Input: part model. Units: mm. Frame: model coordinates. A direction names the side the tool comes from. Coordinates: 2 decimals unless noted, no trailing zeros. Write each loop counter-clockwise with the first axis right and the second up, starting at its lowest first coordinate (ties: lowest second). Pieces come first, ordered by that corner, then holes. Notation, with made-up numbers: (39.25, -34) - (93.25, -34) arc R19 ccw to (93.25, 2) - close; hole circle Ø8 at (15.25, 9.5). An arc over 180 degrees is marked (long way). One line per question, with ' | ' between items. Start each with the question number.
1) Section query C-C on x = -17. Return loops of the section in (y, z), and give its area (3 significant figures).
2) First-contact query: P1, Ø14.5, axis at y = -453, z = 0, coming from the +X side. Flat tip, straight axial feed; report the tip coordinate or a pass-through.
3) Section query B-B on y = -453. Return loops of the section in (x, z), and give its area (3 significant figures).
4) Draft query along Y for faces 1 (the cylindrical face through (-28.986, -444.686, -3.447)), 2 (the flat face through (2, 0, -29)), 3 (the flat face through (0, -232, -30)), 4 (the cylindrical face through (28.986, -444.686, 3.447)). Return one class per face: released by +Y, released by -Y, zero draft, split by the parting line, or undercut.
5) Section query A-A on z = -23. Return loops of the section in (x, y).
6) Line query: line 1 (X direction, y = -154, z = 12.5); line 2 (Z direction, x = -29.2, y = -453); line 3 (Y direction, x = 28.55, z = 0). Output: solid intervals per line, ascending.
7) Reachability of faces 5 (the flat face through (28, -232, 0)), 6 (the flat face through (30, -232, 0)) from +Z, -Z, +X, -X, +Y, -Y: full face, straight path, thin tool, end or side. Return the list, or none.
8) Section query D-D on y = -239. Return loops of the section in (x, z), and give its area (3 significant figures).
Autodesk Inventor part; units mm, degrees
ref_plane "YZ Plane" through (0, 0, 0) normal (1, 0, 0) x (0, 1, 0)
ref_plane "XZ Plane" through (0, 0, 0) normal (0, 1, 0) x (-1, 0, 0)
ref_plane "XY Plane" through (0, 0, 0) normal (0, 0, 1) x (1, 0, 0)
sketch "Sketch9" plane through (0, 0, 0) normal (0, 1, 0) x (-1, 0, 0)
  line L0 (30, 30) -> (-30, 30)
  line L1 (-30, 30) -> (-30, -30)
  line L2 (-30, -30) -> (30, -30)
  line L3 (30, -30) -> (30, 30)
  line L4 (30, 30) -> (-30, -30) construction
  line L5 (-30, 30) -> (30, -30) construction
  line L6 (-28, 28) -> (28, 28)
  line L7 (28, 28) -> (28, -28)
  line L8 (28, -28) -> (-28, -28)
  line L9 (-28, -28) -> (-28, 28)
  point P0 (0, 0)
  dimension "d172" = 60
  dimension "d173" = 60
  dimension "d174" = 2
extrude "Extrusion3" add sketch "Sketch9" against normal blind 470
sketch "Sketch10" plane through (0, 0, 0) normal (1, 0, 0) x (0, 1, 0)
  line L0 (0, 30) -> (0, -30) construction
  line L1 (0, 30) -> (-470, 30) construction
  line L2 (-470, -30) -> (-470, 30) construction
  line L3 (0, -30) -> (-470, -30) construction
  line L4 (-58.25, 15.25) -> (-27.75, 15.25)
  line L5 (-27.75, 15.25) -> (-27.75, -15.25)
  line L6 (-27.75, -15.25) -> (-58.25, -15.25)
  line L7 (-58.25, -15.25) -> (-58.25, 15.25)
  line L8 (-58.25, 15.25) -> (-27.75, -15.25) construction
  line L9 (-27.75, 15.25) -> (-58.25, -15.25) construction
  line L10 (-218.25, 15.25) -> (-187.75, 15.25)
  line L11 (-187.75, 15.25) -> (-187.75, -15.25)
  line L12 (-187.75, -15.25) -> (-218.25, -15.25)
  line L13 (-218.25, -15.25) -> (-218.25, 15.25)
  line L14 (-218.25, 15.25) -> (-187.75, -15.25) construction
  line L15 (-187.75, 15.25) -> (-218.25, -15.25) construction
  line L16 (-368.25, 15.25) -> (-337.75, 15.25)
  line L17 (-337.75, 15.25) -> (-337.75, -15.25)
  line L18 (-337.75, -15.25) -> (-368.25, -15.25)
  line L19 (-368.25, -15.25) -> (-368.25, 15.25)
  line L20 (-368.25, 15.25) -> (-337.75, -15.25) construction
  line L21 (-337.75, 15.25) -> (-368.25, -15.25) construction
  circle A0 centre (-453, 0) radius 9
  line L22 (0, 0) -> (47, 0)
  point P0 (-43, 0)
  point P1 (-203, 0)
  point P2 (-353, 0)
  dimension "d177" = 30.5
  dimension "d178" = 30.5
  dimension "d181" = 47
  dimension "d182" = 90
  dimension "d183" = 250
  dimension "d184" = 400
  dimension "d185" = 500
  dimension "d186" = 18
extrude "Extrusion4" cut sketch "Sketch10" along normal through all both and the other way through all
sketch "Sketch11" plane through (30, 0, 30) normal (1, 0, 0) x (0, 0, -1)
  line L0 (45.25, -218.25) -> (14.75, -218.25)
  line L1 (14.75, -218.25) -> (14.75, -187.75)
  line L2 (14.75, -187.75) -> (45.25, -187.75)
  line L3 (45.25, -187.75) -> (45.25, -218.25)
  circle A0 centre (30, -453) radius 9
  line L4 (45.25, -58.25) -> (14.75, -58.25)
  line L5 (14.75, -58.25) -> (14.75, -27.75)
  line L6 (14.75, -27.75) -> (45.25, -27.75)
  line L7 (45.25, -27.75) -> (45.25, -58.25)
  line L8 (45.25, -368.25) -> (14.75, -368.25)
  line L9 (14.75, -368.25) -> (14.75, -337.75)
  line L10 (14.75, -337.75) -> (45.25, -337.75)
  line L11 (45.25, -337.75) -> (45.25, -368.25)
  line L12 (0, 0) -> (60, 0)
  line L13 (0, 0) -> (0, -470)
  line L14 (60, -470) -> (0, -470)
  line L15 (60, 0) -> (60, -470)
  line L16 (45.25, -27.75) -> (14.75, -58.25)
  line L17 (45.25, -187.75) -> (14.75, -218.25)
  line L18 (45.25, -337.75) -> (14.75, -368.25)
  point P0 (30, 0)
sketch "Sketch13" plane through (-30, 0, -30) normal (-1, 0, 0) x (0, 0, 1)
  line L0 (45.25, -218.25) -> (14.75, -218.25)
  line L1 (14.75, -218.25) -> (14.75, -187.75)
  line L2 (14.75, -187.75) -> (45.25, -187.75)
  line L3 (45.25, -187.75) -> (45.25, -218.25)
  circle A0 centre (30, -453) radius 9
  line L4 (45.25, -58.25) -> (14.75, -58.25)
  line L5 (14.75, -58.25) -> (14.75, -27.75)
  line L6 (14.75, -27.75) -> (45.25, -27.75)
  line L7 (45.25, -27.75) -> (45.25, -58.25)
  line L8 (45.25, -368.25) -> (14.75, -368.25)
  line L9 (14.75, -368.25) -> (14.75, -337.75)
  line L10 (14.75, -337.75) -> (45.25, -337.75)
  line L11 (45.25, -337.75) -> (45.25, -368.25)
  line L12 (0, 0) -> (60, 0)
  line L13 (0, 0) -> (0, -470)
  line L14 (60, -470) -> (0, -470)
  line L15 (60, 0) -> (60, -470)
  line L16 (14.75, -58.25) -> (45.25, -27.75)
  line L17 (14.75, -218.25) -> (45.25, -187.75)
  line L18 (14.75, -368.25) -> (45.25, -337.75)
  point P0 (30, 0)
fillet "Fillet1" radius 2 24 edges at (29, -337.75, -15.25) (29, -337.75, 15.25) (29, -368.25, 15.25) (29, -368.25, -15.25) (29, -218.25, -15.25) (29, -218.25, 15.25) (29, -187.75, 15.25) (29, -187.75, -15.25) (29, -58.25, 15.25) (29, -27.75, 15.25) (29, -27.75, -15.25) (29, -58.25, -15.25) (-29, -58.25, 15.25) (-29, -27.75, 15.25) (-29, -27.75, -15.25) (-29, -58.25, -15.25) (-29, -187.75, 15.25) (-29, -218.25, 15.25) (-29, -218.25, -15.25) (-29, -187.75, -15.25) (-29, -337.75, 15.25) (-29, -368.25, 15.25) (-29, -337.75, -15.25) (-29, -368.25, -15.25)
properties part number "TZS 753 FDS 1200 FLANGE 3" material "Stainless Steel"
Answer key:
1) outline: (-470, -30) - (0, -30) - (0, -28) - (-470, -28) - close; (-470, 28) - (0, 28) - (0, 30) - (-470, 30) - close | area: 1,880 mm²
2) P1: through
3) outline: (-30, -30) - (30, -30) - (30, -9) - (28, -9) - (28, -28) - (-28, -28) - (-28, -9) - (-30, -9) - close; (-30, 9) - (-28, 9) - (-28, 28) - (28, 28) - (28, 9) - (30, 9) - (30, 30) - (-30, 30) - close | area: 392 mm²
4) face 1: undercut | face 2: released by +Y | face 3: zero draft | face 4: undercut
5) outline: (-30, -470) - (-28, -470) - (-28, 0) - (-30, 0) - close; (28, -470) - (30, -470) - (30, 0) - (28, 0) - close
6) line 1: -30 to -28, 28 to 30 | line 2: -30 to -9, 9 to 30 | line 3: -470 to -462, -444 to -368.25, -337.75 to -218.25, -187.75 to -58.25, -27.75 to 0
7) face 5: +Y, -Y | face 6: +Z, -Z, +X, +Y, -Y
8) outline: (-30, -30) - (30, -30) - (30, 30) - (-30, 30) - close; hole (-28, -28) - (28, -28) - (28, 28) - (-28, 28) - close | area: 464 mm²
